Build history of the part. All positions in model axes, mm. Face numbers are marked on the shaded views. A direction names the side the tool comes from. Round coordinates to 2 decimals unless told otherwise and drop trailing zeros. Write each loop counter-clockwise with the first axis right and the second up, starting at its lowest first coordinate (ties: lowest second). Pieces come first, ordered by that corner, then holes.
from build123d import *

# Parameters (mm, degrees)
F0_R     = 3
F0_R_2   = 2.3
F1_DEPTH = 5
F3_START = -2.5
F2_W     = 6
F2_H     = 5
F3_DEPTH = 0.5


with BuildPart() as f1:
    # F0 (on Front) → F1 (new body)
    with BuildSketch(Plane.XZ):
        Circle(F0_R)
        Circle(F0_R_2, mode=Mode.SUBTRACT)
    extrude(amount=F1_DEPTH)

    # F2 (on Top) → F3 (join)
    with BuildSketch(Plane.XY.offset(F3_START)):
        with Locations((0, -2.5)):
            Rectangle(F2_W, F2_H)
    extrude(amount=-F3_DEPTH)


solid = f1.part
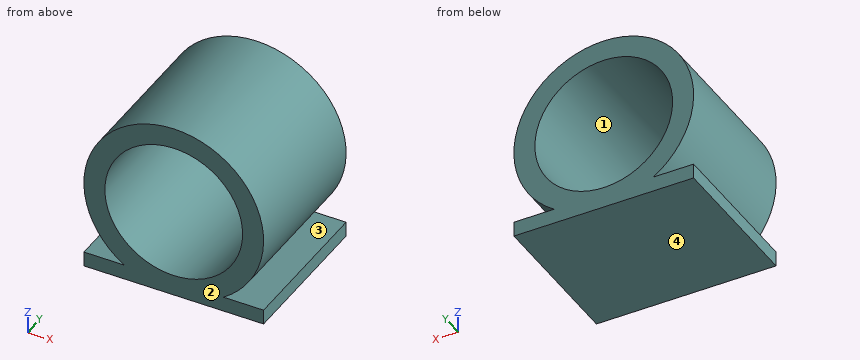
1) Slice it at A-A (x = 0). Write the cut outline in (y, z).
Results:
outline: (-5, -3) - (0, -3) - (0, -2.3) - (-5, -2.3) - close; (-5, 2.3) - (0, 2.3) - (0, 3) - (-5, 3) - close
2) Which spindle directions (+Z, -Z, +X, -X, +Y, -Y) get a long thin tool onto all of the face, cutting with end or side? Do the marked faces 3 and 4. Say none if no direction does.
Results:
face 3: +X, +Y, -Y
face 4: -Z, +X, -X, +Y, -Y
3) Wall check: L1, parallel to Z at x = 0, y = -2.9; L2, parallel to Z at x = -2, y = -3.8; L3, parallel to X at y = -1.7, z = -1.55. Give the ranges that are in metal, low to high.
Results:
L1: z = -3 to -2.3, 2.3 to 3
L2: z = -3 to -2.5, -2.24 to -1.14, 1.14 to 2.24
L3: x = -2.57 to -1.7, 1.7 to 2.57
4) Slice it at B-B (z = 0). Write the cut outline in (x, y), plus the area to 3 significant figures.
Results:
outline: (-3, -5) - (-2.3, -5) - (-2.3, 0) - (-3, 0) - close; (2.3, -5) - (3, -5) - (3, 0) - (2.3, 0) - close
area: 7.00 mm2
5) Slice it at D-D (z = 2.6). Write the cut outline in (x, y), plus the area to 3 significant figures.
Results:
outline: (-1.5, -5) - (1.5, -5) - (1.5, 0) - (-1.5, 0) - close
area: 15.0 mm2
6) Pin check, flat tips, straight feed: pin 1 Ø1 at (y, z) = (-4, -1) entering from -X; pin 2 Ø1.1 at (x, y) = (-2.5, -3) entering from +Z; pin 3 Ø2 at (x, z) = (1, 1) entering from -Y; pin 4 Ø1.5 at (y, z) = (-1, 2) entering from +X. Stop position of each tip, or through.
Results:
pin 1: stops at x = -2.96
pin 2: stops at z = 2.28
pin 3: stops at y = -5
pin 4: stops at x = 2.73
7) Slice it at C-C (y = -3.7). Write the cut outline in (x, z).
Results:
outline: (-3, -3) - (3, -3) - (3, -2.5) - (1.66, -2.5) arc R3 ccw (long way) to (-1.66, -2.5) - (-3, -2.5) - close; hole circle Ø4.6 at (0, 0)
8) Mould opens along X. For the marked faces 1 and 2 say: released by +X, released by -X, zero draft, split by the parting line, or undercut.
Results:
face 1: undercut
face 2: zero draft
